Can you work these out from the model? Positions are in its coordinate system, mm. Give positions to 0.01 mm unless a question says otherwise; leave off trailing zeros. Order: outer loops, then holes, each group sorted by start corner. A loop starts at its lowest first (then second) coordinate and runs counter-clockwise, first axis right, second up. Notation, with made-up numbers: (5, -29.75) - (37, -29.75) arc R29 cw to (37, -4.75) - close; hole circle Ø4 at (87.25, 49). An arc over 180 degrees is marked (long way). Answer as a JSON object with one key per item and string values.
Autodesk Inventor part; units mm, degrees
ref_plane "YZ Plane" through (0, 0, 0) normal (1, 0, 0) x (0, 1, 0)
ref_plane "XZ Plane" through (0, 0, 0) normal (0, 1, 0) x (-1, 0, 0)
ref_plane "XY Plane" through (0, 0, 0) normal (0, 0, 1) x (1, 0, 0)
sketch "Sketch1" plane through (0, 0, 0) normal (0, 0, 1) x (1, 0, 0)
  line L0 (-130, 67.5) -> (-130, -67.5)
  line L1 (-130, -67.5) -> (-120, -67.5)
  line L2 (-120, -67.5) -> (-120, -70)
  line L3 (-120, -70) -> (120, -70)
  line L4 (120, -70) -> (120, -67.5)
  line L5 (120, -67.5) -> (130, -67.5)
  line L6 (130, -67.5) -> (130, 67.5)
  line L7 (130, 67.5) -> (120, 67.5)
  line L8 (120, 67.5) -> (120, 72.5)
  line L9 (120, 72.5) -> (-120, 72.5)
  line L10 (-120, 72.5) -> (-120, 67.5)
  line L11 (-130, 67.5) -> (-120, 67.5)
  point P0 (0, 0)
  point P1 (0, 72.5)
  point P2 (130, 0)
  point P3 (-130, 0)
  dimension "d0" = 5
  dimension "d1" = 240
  dimension "d2" = 10
  dimension "d3" = 10
  dimension "d4" = 2.5
  dimension "d5" = 135
extrude "Extrusion1" add sketch "Sketch1" along normal blind 5
sketch "Sketch2" plane through (0, 0, 5) normal (0, 0, 1) x (1, 0, 0)
  line L0 (25, -15.75) -> (52.5, -15.75)
  line L1 (52.5, -15.75) -> (52.5, 15.75)
  line L2 (52.5, 15.75) -> (25, 15.75)
  line L3 (25, 15.75) -> (25, -15.75)
  line L4 (77.5, -15.75) -> (105, -15.75)
  line L5 (105, -15.75) -> (105, 15.75)
  line L6 (105, 15.75) -> (77.5, 15.75)
  line L7 (77.5, 15.75) -> (77.5, -15.75)
  line L8 (130, -67.5) -> (130, 67.5)
  point P0 (0, 0)
  point P1 (25, 0)
  point P2 (77.5, 0)
  dimension "d8" = 27.5
  dimension "d9" = 31.5
  dimension "d10" = 27.5
  dimension "d11" = 31.5
  dimension "d12" = 130
  dimension "d13" = 25
  dimension "d14" = 25
extrude "Extrusion2" cut sketch "Sketch2" against normal through all
sketch "Sketch3" plane through (0, 0, 5) normal (0, 0, 1) x (1, 0, 0)
  line L0 (20.75, 0) -> (56.75, 0) construction
  line L1 (25, 15.75) -> (52.5, 15.75)
  line L2 (77.5, 15.75) -> (105, 15.75)
  line L3 (73.25, 0) -> (109.25, 0) construction
  point P0 (0, 0)
  point P1 (38.75, 0)
  point P2 (38.75, 15.75)
  point P3 (91.25, 0)
  point P4 (91.25, 15.75)
  dimension "d17" = 36
  dimension "d18" = 36
hole "Hole1" at (20.75, 0, 5) at (56.75, 0, 5) at (73.25, 0, 5) at (109.25, 0, 5) direction (0, 0, -1) diameter 3.4 depth 8 tip angle 118
fillet "Fillet1" radius 2.5 8 edges at (25, 15.75, 2.5) (77.5, 15.75, 2.5) (105, 15.75, 2.5) (52.5, 15.75, 2.5) (52.5, -15.75, 2.5) (105, -15.75, 2.5) (25, -15.75, 2.5) (77.5, -15.75, 2.5)
sketch "Sketch5" plane through (0, 0, 5) normal (0, 0, 1) x (1, 0, 0)
  circle A0 centre (-94, 0) radius 32
  circle A1 centre (-26, 0) radius 32
  line L0 (-130, 67.5) -> (-130, -67.5)
  point P0 (0, 0)
  dimension "d34" = 64
  dimension "d35" = 68
  dimension "d36" = 36
  dimension "d37" = 64
extrude "Extrusion3" cut sketch "Sketch5" against normal through all
sketch "Sketch6" plane through (0, 0, 5) normal (0, 0, 1) x (1, 0, 0)
  point P0 (0, 0)
  point P1 (65, -40)
  dimension "d40" = 65
  dimension "d60" = 40
hole "Hole3" at (65, -40, 5) direction (0, 0, -1) diameter 6.6 depth 8 tip angle 118
sketch "Sketch7" plane through (0, 0, 5) normal (0, 0, 1) x (1, 0, 0)
  circle A0 centre (-94, 0) radius 32 construction
  circle A1 centre (-26, 0) radius 32 construction
  line L0 (-117.5, -30) -> (-2.5, -30) construction
  line L1 (-2.5, -30) -> (-2.5, 30) construction
  line L2 (-2.5, 30) -> (-117.5, 30) construction
  line L3 (-117.5, 30) -> (-117.5, -30) construction
  line L4 (-117.5, -30) -> (-2.5, 30) construction
  line L5 (-2.5, -30) -> (-117.5, 30) construction
  point P0 (0, 0)
  point P1 (-60, 0)
  point P2 (-60, 0)
  dimension "d49" = 68
  dimension "d50" = 34
  dimension "d51" = 115
  dimension "d52" = 60
hole "Hole4" at (-117.5, 30, 5) at (-117.5, -30, 5) at (-2.5, -30, 5) at (-2.5, 30, 5) direction (0, 0, -1) diameter 5.5 depth 8 tip angle 118
sketch "Sketch8" plane through (0, 0, 5) normal (0, 0, 1) x (1, 0, 0)
  circle A0 centre (65, -40) radius 3.3 construction
  line L0 (65, 58.5) -> (65, 21.5) construction
  point P0 (0, 0)
  point P1 (65, 40)
  dimension "d62" = 37
  dimension "d63" = 40
  dimension "d71" = 0
hole "Hole5" at (65, 21.5, 5) at (65, 58.5, 5) direction (0, 0, -1) diameter 3.4 depth 8 tip angle 118
equation "\"d14\" = d13"
properties part number "SeitenOben" material "Polycarbonate, Clear"
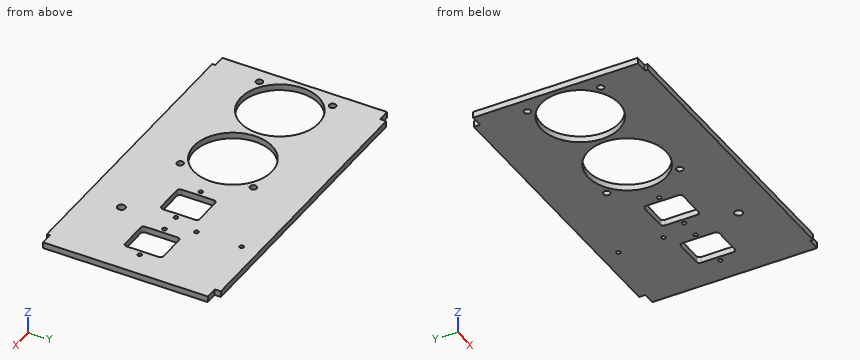
Q1. I'm going to push flat-ended pins straight in: pin 1 Ø2.5 at (x, y) = (109.25, 0) entering from -Z; pin 2 Ø0.8 at (y, z) = (-69, 1.5) entering from +X. Where does each tip first touch, or does it pass through?
Recorded:
{"pin 1": "passes through", "pin 2": "stops at x = 120"}
Q2. I need wall thicknesses on L1, parallel to Y at x = 65, z = 3.8; L2, parallel to Y at x = 109.5, z = 3.3; L3, parallel to X at y = 29.5, z = 1.7. Which ranges of each line are inside material? Lowest first, please.
Recorded:
{"L1": "y = -70 to -43.3, -36.7 to 19.8, 23.2 to 56.8, 60.2 to 72.5", "L2": "y = -70 to -1.68, 1.68 to 72.5", "L3": "x = -130 to -120.2, -114.8 to -106.4, -81.6 to -38.4, -13.6 to -5.2, 0.2 to 130"}
Q3. If we section it at D-D, the plane z = 0.8: Count the separate pieces of the cut face and the enclosed holes in it, then the cut area to 3 significant figures.
Recorded:
{"separate pieces": "1", "enclosed holes": "15", "area": "28,600 mm^2"}
Q4. If we section it at B-B, the plane y = 7.5: Please give me the cut outline in (x, z).
Recorded:
{"outline": "(-130, 0) - (-125.11, 0) - (-125.11, 5) - (-130, 5) - close; (-62.89, 0) - (-57.11, 0) - (-57.11, 5) - (-62.89, 5) - close; (5.11, 0) - (25, 0) - (25, 5) - (5.11, 5) - close; (52.5, 0) - (77.5, 0) - (77.5, 5) - (52.5, 5) - close; (105, 0) - (130, 0) - (130, 5) - (105, 5) - close"}
Q5. If we section it at A-A, the plane x = 44.5: Please give me the cut outline in (y, z), then the cut area to 3 significant figures.
Recorded:
{"outline": "(-70, 0) - (-15.75, 0) - (-15.75, 5) - (-70, 5) - close; (15.75, 0) - (72.5, 0) - (72.5, 5) - (15.75, 5) - close", "area": "555 mm^2"}
Q6. If we section it at C-C, the plane x = -2.5: Please give me the cut outline in (y, z).
Recorded:
{"outline": "(-70, 0) - (-32.75, 0) - (-32.75, 5) - (-70, 5) - close; (-27.25, 0) - (-21.72, 0) - (-21.72, 5) - (-27.25, 5) - close; (21.72, 0) - (27.25, 0) - (27.25, 5) - (21.72, 5) - close; (32.75, 0) - (72.5, 0) - (72.5, 5) - (32.75, 5) - close"}
